Part model, mm, in its own coordinate system. Face numbers are marked on the shaded views. A direction names the side the tool comes from. Coordinates: 2 decimals unless noted, no trailing zeros. Write each loop counter-clockwise with the first axis right and the second up, starting at its lowest first coordinate (ties: lowest second). Pieces come first, ordered by that corner, then holes. Notation, with made-up numbers: (53, 41) - (102, 41) arc R20 cw to (102, 63) - close; hole circle Ø7 at (14.5, 22.25). An arc over 180 degrees is marked (long way). Write each question's results on one line, items separated by ' | '.
from build123d import *

# Parameters (mm, degrees)
F0_W     = 203.2
F0_H     = 101.6
F1_DEPTH = 304.8
F2_W     = 101.6
F2_H     = 69.85
F3_DEPTH = 203.201
F4_R     = 7.62


with BuildPart() as f1:
    # F0 (on Front) → F1 (new body)
    with BuildSketch(Plane.XZ):
        Rectangle(F0_W, F0_H)
    extrude(amount=F1_DEPTH)

    # F2 (on face) → F3 (cut, through all)
    with BuildSketch(Plane.YZ.offset(101.6)):
        with Locations((-228.6, 0)):
            Rectangle(F2_W, F2_H)
        with Locations((-76.2, 0)):
            Rectangle(F2_W, F2_H)
    extrude(amount=-F3_DEPTH, mode=Mode.SUBTRACT)

    # F4
    f4_edges = [f1.edges().sort_by_distance(p)[0] for p in [
        (-101.6, -152.4, 50.8),
        (-101.6, 0, 0),
        (-101.6, -304.8, 0),
        (-101.6, -152.4, -50.8),
        (-101.6, -177.8, 0),
        (-101.6, -228.6, 34.925),
        (-101.6, -279.4, 0),
        (-101.6, -228.6, -34.925),
        (-101.6, -25.4, 0),
        (-101.6, -76.2, 34.925),
        (-101.6, -127, 0),
        (-101.6, -76.2, -34.925),
        (101.6, -152.4, -50.8),
        (101.6, 0, 0),
        (101.6, -304.8, 0),
        (101.6, -152.4, 50.8),
        (101.6, -228.6, -34.925),
        (101.6, -279.4, 0),
        (101.6, -228.6, 34.925),
        (101.6, -177.8, 0),
        (101.6, -76.2, -34.925),
        (101.6, -127, 0),
        (101.6, -76.2, 34.925),
        (101.6, -25.4, 0),
    ]]
    fillet(f4_edges, radius=F4_R)


solid = f1.part
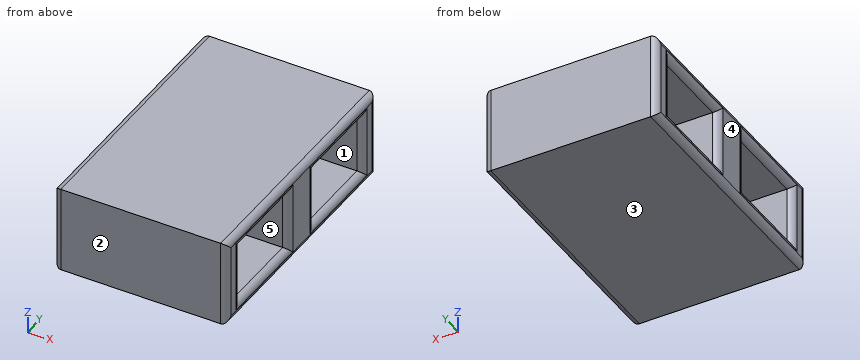
(1) 3-axis set-ups, long thin cutter, end or side, ignore diameter. For the marked faces 4 and 5: which of +Z, -Z, +X, -X, +Y, -Y reach the whole face in a straight line?
Return value:
face 4: +Z, -Z, -X, +Y, -Y | face 5: +X, -X
(2) Two-plate mould, pull along Y, no slides. Class the marked faces 1, 2 and 3: released by +Y, released by -Y, zero draft, split by the parting line, or undercut.
Return value:
face 1: undercut | face 2: released by -Y | face 3: zero draft
(3) Wall check: line 1 (Y direction, x = 81, z = -15); line 2 (Z direction, x = 8.5, y = -237) (3 decimals); line 3 (X direction, y = -93.5, z = -42). Give the ranges that are in metal, low to high. Write a range as from..to.
Return value:
line 1: y = -304.8..-279.4, -177.8..-127, -25.4..0 | line 2: z = -50.8..-34.925, 34.925..50.8 | line 3: x = -101.58..101.58
(4) Saw through at C-C on x = 51. Write the cut outline in (y, z) (3 decimals), then the cut area to 3 significant figures.
Return value:
outline: (-304.8, -50.8) - (0, -50.8) - (0, 50.8) - (-304.8, 50.8) - close; hole (-279.4, -34.925) - (-177.8, -34.925) - (-177.8, 34.925) - (-279.4, 34.925) - close; hole (-127, -34.925) - (-25.4, -34.925) - (-25.4, 34.925) - (-127, 34.925) - close | area: 16,800 mm^2
(5) Saw through at A-A on z = 30.5. Write the cut outline in (x, y), then the cut area to 3 significant figures.
Return value:
outline: (-101.6, -297.18) arc R7.62 ccw to (-93.98, -304.8) - (93.98, -304.8) arc R7.62 ccw to (101.6, -297.18) - (101.6, -287.02) arc R7.62 ccw to (93.98, -279.4) - (-93.98, -279.4) arc R7.62 ccw to (-101.6, -287.02) - close; (-101.6, -170.18) arc R7.62 ccw to (-93.98, -177.8) - (93.98, -177.8) arc R7.62 ccw to (101.6, -170.18) - (101.6, -134.62) arc R7.62 ccw to (93.98, -127) - (-93.98, -127) arc R7.62 ccw to (-101.6, -134.62) - close; (-101.6, -17.78) arc R7.62 ccw to (-93.98, -25.4) - (93.98, -25.4) arc R7.62 ccw to (101.6, -17.78) - (101.6, -7.62) arc R7.62 ccw to (93.98, 0) - (-93.98, 0) arc R7.62 ccw to (-101.6, -7.62) - close | area: 20,500 mm^2
(6) Saw through at B-B on y = -238. Write the cut outline in (x, z) (3 decimals).
Return value:
outline: (-101.6, -43.18) arc R7.62 ccw to (-93.98, -50.8) - (93.98, -50.8) arc R7.62 ccw to (101.6, -43.18) - (101.6, -42.545) arc R7.62 ccw to (93.98, -34.925) - (-93.98, -34.925) arc R7.62 ccw to (-101.6, -42.545) - close; (-101.6, 42.545) arc R7.62 ccw to (-93.98, 34.925) - (93.98, 34.925) arc R7.62 ccw to (101.6, 42.545) - (101.6, 43.18) arc R7.62 ccw to (93.98, 50.8) - (-93.98, 50.8) arc R7.62 ccw to (-101.6, 43.18) - close
